Drawing for the job (mm, zero at the part's lowest x, y, z). A direction names the side the tool comes from. Coordinates: 2 decimals unless noted, no trailing zeros. Write each loop counter-clockwise with the first axis right and the second up, starting at its lowest first coordinate (ties: lowest second). Pieces come first, ordered by that corner, then holes. Notation, with made-up numbers: M -6.5,86.5 L 13.5,86.5 A10 ccw 13.5,92.5 Z; hole C -35.75,17 d2. An arc over 180 degrees is marked long. Put each result on its own line as item: value. Start each with the question number.
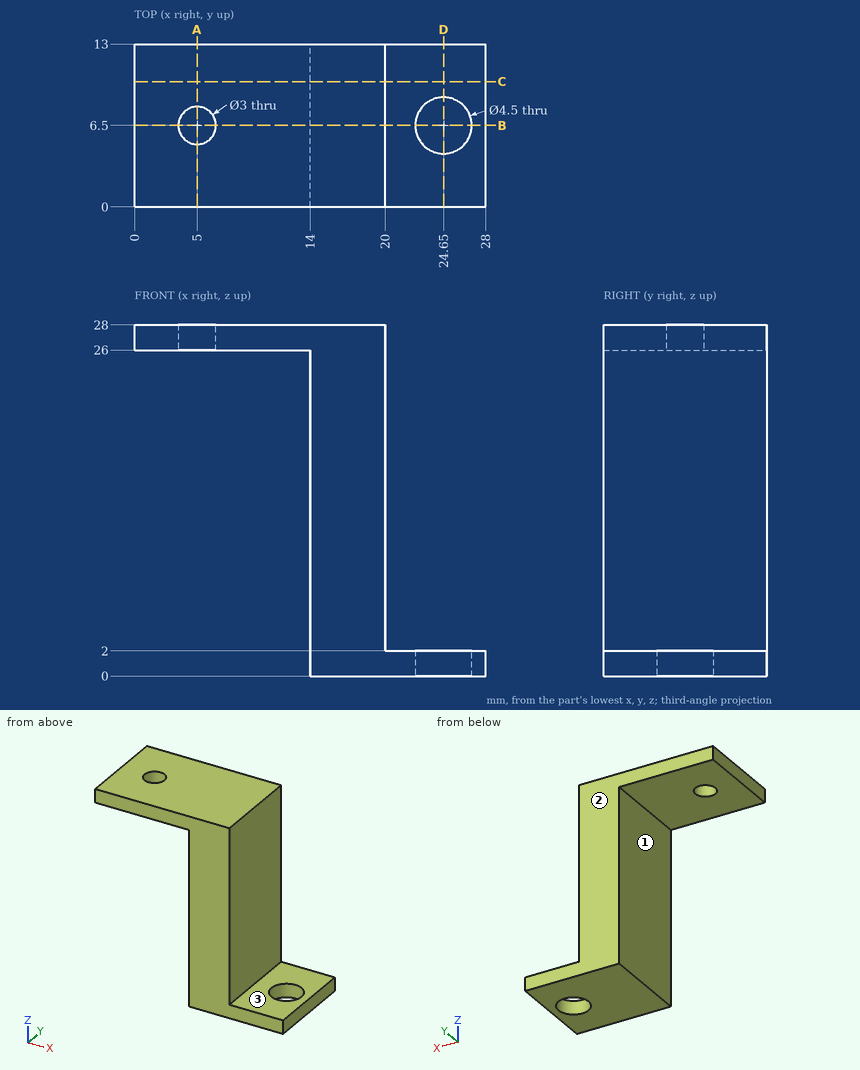
(1) Slice it at D-D, the plane x = 24.65. Write the cut outline in (y, z), then the cut area to 3 significant figures.
(2) Which spindle directions (+Z, -Z, +X, -X, +Y, -Y) get a long thin tool onto all of the face, cutting with end or side? Do the marked faces 1, 2 and 3. Say none if no direction does.
(3) Drop flat-ended pins along their axis: pin 1 (4 mm diameter, centred on x = 4, y = 8.5, fed in from -Z); pin 2 (5 mm diameter, centred on x = 24.65, y = 6.5, fed in from +Z); pin 3 (5 mm diameter, centred on x = 16.5, z = 5.5, fed in from -Y); pin 4 (4 mm diameter, centred on y = 4, z = 11, fed in from -X). Give the stop position or say it passes through.
(4) Slice it at B-B, the plane y = 6.5. Write the cut outline in (x, z).
(5) Slice it at C-C, the plane y = 10. Write the cut outline in (x, z).
(6) Slice it at A-A, the plane x = 5. Write the cut outline in (y, z), then the cut area to 3 significant figures.
(7) Drill centre lines: line 1 (Y direction, x = 5, z = 26.65); line 2 (Y direction, x = 24.65, z = 0.6); line 3 (Z direction, x = 1.5, y = 1.5). Where is each one in solid material? Low to high. Write a range as [from, to].
Result set:
1. outline: M 0,0 L 4.25,0 L 4.25,2 L 0,2 Z; M 8.75,0 L 13,0 L 13,2 L 8.75,2 Z
1. area: 17.0 mm^2
2. face 1: -Z, -X, +Y, -Y
2. face 2: +Z, -Z, +X, -X, +Y
2. face 3: +Z, +X, +Y, -Y
3. pin 1: stops at z = 26
3. pin 2: stops at z = 2
3. pin 3: stops at y = 0
3. pin 4: stops at x = 14
4. outline: M 0,26 L 3.5,26 L 3.5,28 L 0,28 Z; M 6.5,26 L 14,26 L 14,0 L 22.4,0 L 22.4,2 L 20,2 L 20,28 L 6.5,28 Z; M 26.9,0 L 28,0 L 28,2 L 26.9,2 Z
5. outline: M 0,26 L 14,26 L 14,0 L 28,0 L 28,2 L 20,2 L 20,28 L 0,28 Z
6. outline: M 0,26 L 5,26 L 5,28 L 0,28 Z; M 8,26 L 13,26 L 13,28 L 8,28 Z
6. area: 20.0 mm^2
7. line 1: y = [0, 5], [8, 13]
7. line 2: y = [0, 4.25], [8.75, 13]
7. line 3: z = [26, 28]
